Could you check a few things on this model? Use its own coordinates, in mm. A direction names the side the tool comes from. Round coordinates to 2 decimals unless told otherwise and drop trailing zeros. Loops run counter-clockwise (first coordinate to the right, second up) from the corner with the lowest first, then second, coordinate; pieces in that order, holes last.
from build123d import *

# Parameters (mm, degrees)
CROQUIS1_W               = 5.98
CROQUIS1_H               = 2.26
CROQUIS1_R               = 1
SALIENTE_EXTRUIR1_DEPTH  = 3.2
CROQUIS2_W               = 2.18
CROQUIS2_H               = 0.38
SALIENTE_EXTRUIR2_DEPTH  = 3.2
CROQUIS4_W               = 1.68598805
CROQUIS4_H               = 3.2
SALIENTE_EXTRUIR3_DEPTH  = 5.5
SALIENTE_EXTRUIR4_DEPTH  = 3.2
REDONDEO2_R              = 0.3
REDONDEO3_R              = 0.21
CROQUIS6_W               = 3.2
CROQUIS6_H               = 7.76
SALIENTE_EXTRUIR5_DEPTH  = 0.5
CROQUIS7_W               = 2.18598805
CROQUIS7_H               = 7.76
SALIENTE_EXTRUIR6_DEPTH  = 1.6
SALIENTE_EXTRUIR7_START  = 1.6
SALIENTE_EXTRUIR7_DEPTH  = 1.6
CORTAR_EXTRUIR2_START    = -10
CORTAR_EXTRUIR2_DEPTH    = 10
CROQUIS11_W              = 4.8
CROQUIS11_H              = 2.64
SALIENTE_EXTRUIR8_DEPTH  = 1
CROQUIS15_W              = 4.3
CROQUIS15_H              = 4.8
SALIENTE_EXTRUIR10_DEPTH = 0.38
REDONDEO6_R              = 3.2
CROQUIS16_W              = 5.29401195
CROQUIS16_H              = 4.8
SALIENTE_EXTRUIR11_DEPTH = 0.4
SALIENTE_EXTRUIR12_START = 0.8
CROQUIS18_R              = 1
SALIENTE_EXTRUIR12_DEPTH = 0.8
REDONDEO7_R              = 0.5
CROQUIS19_W              = 4.2
CROQUIS19_H              = 1.2
CORTAR_EXTRUIR3_DEPTH    = 3
SALIENTE_EXTRUIR13_START = -5.6
CROQUIS20_W              = 5.29401195
CROQUIS20_H              = 0.3
SALIENTE_EXTRUIR13_DEPTH = 5.6


with BuildPart() as part:
    # Croquis1 → Saliente-Extruir1 (new body)
    with BuildSketch(Plane.XY):
        Rectangle(CROQUIS1_W, CROQUIS1_H)
        with Locations((-0.44, 0)):
            Circle(CROQUIS1_R, mode=Mode.SUBTRACT)
    extrude(amount=SALIENTE_EXTRUIR1_DEPTH)

    # Croquis2 → Saliente-Extruir2 (add)
    with BuildSketch(Plane.XY):
        with Locations((1.9, -1.32)):
            Rectangle(CROQUIS2_W, CROQUIS2_H)
    extrude(amount=SALIENTE_EXTRUIR2_DEPTH)

    # Croquis4 → Saliente-Extruir3 (add)
    with BuildSketch(Plane(origin=(0, 1.13, 0), x_dir=(1, 0, 0), z_dir=(0, 1, 0))):
        with Locations((-2.147005975, -1.6)):
            Rectangle(CROQUIS4_W, CROQUIS4_H)
    extrude(amount=SALIENTE_EXTRUIR3_DEPTH)

    # Croquis5 → Saliente-Extruir4 (add)
    with BuildSketch(Plane(origin=(0, 0, 0), x_dir=(-1, 0, 0), z_dir=(0, 0, -1))):
        with BuildLine():
            Line((-2.99, -1.51), (-2.312022185, -3.905922804))
            ThreePointArc((-2.312022185, -3.905922804), (-2.072768276, -3.925139809), (-1.86757295, -3.80061429))
            ThreePointArc((-1.86757295, -3.80061429), (-1.807264861, -2.439011425), (-0.81, -1.51))
            Line((-0.81, -1.51), (-2.99, -1.51))
        make_face()
    extrude(amount=-SALIENTE_EXTRUIR4_DEPTH)

    # Redondeo2
    # the kernel refuses this fillet: 0.3 mm, written as the material it takes off along each edge
    with BuildSketch(Plane(origin=(1.86757295, -3.80061429, -1.141887159), x_dir=(0.2702256968555762, 0.9627970049594662, 0), z_dir=(0, 0, 1))) as redondeo2_piece_1:
        with BuildLine():
            CenterArc((0.274279078, -0.299257177), REDONDEO2_R, 94.032824869, 117.548904109)
            Line((0.018710883, -0.456371459), (0.013599519, -0.459513744))
            ThreePointArc((0.013599519, -0.459513744), (-0.07043871, -0.231457229), (-0.005003521, 0.00331131))
            Line((-0.005003521, 0.00331131), (0.000421968, 0.005985144))
            ThreePointArc((0.000421968, 0.005985144), (0.126590344, 0.001543061), (0.25275872, 0.005985144))
            Line((0.25275872, 0.005985144), (0.253180688, 0))
        make_face()
    extrude(amount=5.483774318, mode=Mode.SUBTRACT)

    # Redondeo3
    redondeo3_edges = [part.edges().sort_by_distance(p)[0] for p in [
        (2.312022185, -3.905922804, 1.6),
    ]]
    fillet(redondeo3_edges, radius=REDONDEO3_R)

    # Croquis6 → Saliente-Extruir5 (add)
    with BuildSketch(Plane.ZY.offset(2.99)):
        with Locations((1.6, 2.75)):
            Rectangle(CROQUIS6_W, CROQUIS6_H)
    extrude(amount=SALIENTE_EXTRUIR5_DEPTH)

    # Croquis7 → Saliente-Extruir6 (add)
    with BuildSketch(Plane(origin=(0, 0, 0), x_dir=(-1, 0, 0), z_dir=(0, 0, -1))):
        with Locations((2.397005975, 2.75)):
            Rectangle(CROQUIS7_W, CROQUIS7_H)
    extrude(amount=SALIENTE_EXTRUIR6_DEPTH)

    # Croquis8 → Saliente-Extruir7 (add)
    with BuildSketch(Plane(origin=(0, 0, 0), x_dir=(-1, 0, 0), z_dir=(0, 0, -1)).offset(SALIENTE_EXTRUIR7_START)):
        with BuildLine():
            Line((-0.81, -1.13), (1.30401195, -1.13))
            Line((1.30401195, -1.13), (1.30401195, -0.503471301))
            ThreePointArc((1.30401195, -0.503471301), (-0.56, 0), (1.30401195, 0.503471301))
            Line((1.30401195, 0.503471301), (1.30401195, 1.13))
            Line((1.30401195, 1.13), (-2.99, 1.13))
            Line((-2.99, 1.13), (-2.99, -1.51))
            Line((-2.99, -1.51), (-2.361581826, -3.730782744))
            ThreePointArc((-2.361581826, -3.730782744), (-2.201095129, -3.879446502), (-1.995487215, -3.804731853))
            ThreePointArc((-1.995487215, -3.804731853), (-1.938099887, -3.687426244), (-1.935988878, -3.556852683))
            ThreePointArc((-1.935988878, -3.556852683), (-1.750154515, -2.325947779), (-0.81, -1.51))
            Line((-0.81, -1.51), (-0.81, -1.13))
        make_face()
    extrude(amount=-SALIENTE_EXTRUIR7_DEPTH)

    # Croquis9 → Cortar-Extruir2 (cut)
    with BuildSketch(Plane.XY.offset(CORTAR_EXTRUIR2_START)):
        with BuildLine():
            Line((-1.30401195, -0.503471301), (-1.30401195, 0.503471301))
            ThreePointArc((-1.30401195, 0.503471301), (-1.44, 0), (-1.30401195, -0.503471301))
        make_face()
    extrude(amount=CORTAR_EXTRUIR2_DEPTH, mode=Mode.SUBTRACT)

    # Croquis11 → Saliente-Extruir8 (add)
    with BuildSketch(Plane(origin=(2.99, 0, 0), x_dir=(0, 0, -1), z_dir=(1, 0, 0))):
        with Locations((-0.8, -0.19)):
            Rectangle(CROQUIS11_W, CROQUIS11_H)
    extrude(amount=SALIENTE_EXTRUIR8_DEPTH)

    # Croquis15 → Saliente-Extruir10 (add)
    with BuildSketch(Plane.XZ.offset(1.13)):
        with Locations((-1.34, 0.8)):
            Rectangle(CROQUIS15_W, CROQUIS15_H)
    extrude(amount=SALIENTE_EXTRUIR10_DEPTH)

    # Redondeo6
    redondeo6_edges = [part.edges().sort_by_distance(p)[0] for p in [
        (-3.49, -1.51, 0.8),
    ]]
    fillet(redondeo6_edges, radius=REDONDEO6_R)

    # Croquis16 → Saliente-Extruir11 (add)
    with BuildSketch(Plane(origin=(0, 1.13, 0), x_dir=(1, 0, 0), z_dir=(0, 1, 0))):
        with Locations((1.342994025, -0.8)):
            Rectangle(CROQUIS16_W, CROQUIS16_H)
    extrude(amount=SALIENTE_EXTRUIR11_DEPTH)

    # Croquis18 → Saliente-Extruir12 (add)
    with BuildSketch(Plane(origin=(0, 0, -1.6), x_dir=(-1, 0, 0), z_dir=(0, 0, -1)).offset(SALIENTE_EXTRUIR12_START)):
        with BuildLine():
            Line((-0.81, -1.51), (0.29, -1.51))
            ThreePointArc((0.29, -1.51), (2.5527417, -0.5727417), (3.49, 1.69))
            Line((3.49, 1.69), (3.49, 6.63))
            Line((3.49, 6.63), (1.30401195, 6.63))
            Line((1.30401195, 6.63), (1.30401195, 1.53))
            Line((1.30401195, 1.53), (-3.99, 1.53))
            Line((-3.99, 1.53), (-3.99, -1.51))
            Line((-3.99, -1.51), (-2.99, -1.51))
            Line((-2.99, -1.51), (-2.361581826, -3.730782744))
            ThreePointArc((-2.361581826, -3.730782744), (-2.201095129, -3.879446502), (-1.995487215, -3.804731853))
            ThreePointArc((-1.995487215, -3.804731853), (-1.938099887, -3.687426244), (-1.935988878, -3.556852683))
            ThreePointArc((-1.935988878, -3.556852683), (-1.750154515, -2.325947779), (-0.81, -1.51))
        make_face()
        with Locations((0.44, 0)):
            Circle(CROQUIS18_R, mode=Mode.SUBTRACT)
    extrude(amount=-SALIENTE_EXTRUIR12_DEPTH)

    # Redondeo7
    redondeo7_edges = [part.edges().sort_by_distance(p)[0] for p in [
        (-2.397005975, 6.63, -2.4),
        (-2.397005975, 6.63, 3.2),
        (-1.30401195, 6.63, 0.4),
        (-3.49, 6.63, 0.4),
    ]]
    fillet(redondeo7_edges, radius=REDONDEO7_R)

    # Croquis19 → Cortar-Extruir3 (cut)
    with BuildSketch(Plane(origin=(3.99, 0, 0), x_dir=(0, 0, -1), z_dir=(1, 0, 0))):
        with Locations((-0.4, 0.01)):
            Rectangle(CROQUIS19_W, CROQUIS19_H)
    extrude(amount=-CORTAR_EXTRUIR3_DEPTH, mode=Mode.SUBTRACT)

    # Croquis20 → Saliente-Extruir13 (add)
    with BuildSketch(Plane.XY.offset(3.2).offset(SALIENTE_EXTRUIR13_START)):
        with Locations((1.342994025, 1.68)):
            Rectangle(CROQUIS20_W, CROQUIS20_H)
        with BuildLine():
            Line((-3.49, 1.69), (-3.49, 0.272255312))
            ThreePointArc((-3.49, 0.272255312), (-2.198912464, -1.243607541), (-0.29, -1.81))
            Line((-0.29, -1.81), (1.324488812, -1.81))
            ThreePointArc((1.324488812, -1.81), (1.079738106, -1.63857377), (0.81, -1.51))
            Line((0.81, -1.51), (-0.29, -1.51))
            ThreePointArc((-0.29, -1.51), (-2.5527417, -0.5727417), (-3.49, 1.69))
        make_face()
    extrude(amount=SALIENTE_EXTRUIR13_DEPTH)


solid = part.part
Item 1: If I drill on line 1 along Y through (x, z) = (-0.44, -1.75); line 2 along Y through (x, z) = (3.75, 1.35); line 3 along X through (y, z) = (0, 1.55), over which ranges is the centre line in solid material (lowest first)?
Results list:
line 1: y = -1.81 to -1, 1 to 1.83
line 2: y = -1.51 to -0.59, 0.61 to 1.83
line 3: x = -3.35 to -1.44, 0.56 to 0.99
Item 2: If we section it at C-C, the plane x = -0.44: Please give me the cut outline in (y, z).
Results list:
outline: (-1.81, -2.4) - (-1, -2.4) - (-1, 3.2) - (-1.81, 3.2) - close; (1, -2.4) - (1.83, -2.4) - (1.83, 3.2) - (1, 3.2) - close
Item 3: We'd pull the mould along Y, two halves only. Please class faces 4 (the flat face through (-0.6, 1.2, 3.2)), 5 (the flat face through (3.5, -1.51, 0.4)), 6 (the flat face through (3, 0.61, 0)): released by +Y, released by -Y, zero draft, split by the parting line, or undercut.
Results list:
face 4: zero draft
face 5: released by -Y
face 6: undercut
Item 4: If we section it at B-B, the plane z = 0.9: Please give me the cut outline in (x, y), then the cut area to 3 significant figures.
Results list:
outline: (-3.49, 0.27) arc R3.5 ccw to (-0.29, -1.81) - (1.32, -1.81) arc R1.8 cw to (1.94, -3.56) arc R0.3 ccw to (2, -3.8) arc R0.21 ccw to (2.36, -3.73) - (2.99, -1.51) - (3.99, -1.51) - (3.99, -0.59) - (0.99, -0.59) - (0.99, 0.61) - (3.99, 0.61) - (3.99, 1.83) - (-1.3, 1.83) - (-1.3, 6.13) arc R0.5 ccw to (-1.8, 6.63) - (-2.99, 6.63) arc R0.5 ccw to (-3.49, 6.13) - close; hole circle Ø2 at (-0.44, 0)
area: 30.3 mm2
Item 5: For faces 1 (the flat face through (1, 1.83, 0)), 2 (the flat face through (1, -1.81, 0)), 3 (the flat face through (3, 0, 2.5)), which set-ups out of +Z, -Z, +X, -X, +Y, -Y let a thin tool reach every point of the face, with its end or its side?
Results list:
face 1: +Z, -Z, +X, +Y
face 2: +Z, -Z, -X, -Y
face 3: +X
Item 6: Will these pins go through, and if not, where does the flat tip stop? pin 1 (2 mm diameter, centred on y = 3, z = 1, fed in from +X); pin 2 (2.5 mm diameter, centred on x = 2.5, z = 0, fed in from -Y); pin 3 (0.9 mm diameter, centred on x = 3, z = 0.5, fed in from +Y); pin 4 (0.5 mm diameter, centred on x = 3.5, z = 0.5, fed in from -Y).
Results list:
pin 1: stops at x = -1.3
pin 2: stops at y = -3.88
pin 3: stops at y = 1.83
pin 4: stops at y = -1.51
Item 7: If we section it at A-A, the plane x = 1.75: Please give me the cut outline in (y, z).
Results list:
outline: (-2.33, -2.4) - (1.83, -2.4) - (1.83, 3.2) - (-2.33, 3.2) - close; hole (-0.59, -1.7) - (0.61, -1.7) - (0.61, 2.5) - (-0.59, 2.5) - close
